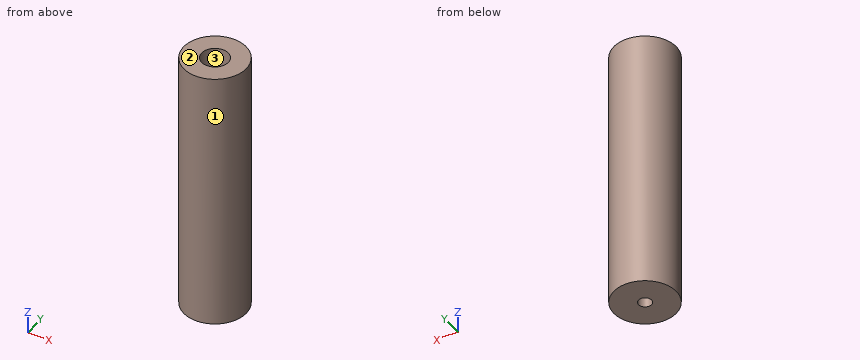
```python
from build123d import *

# Parameters (mm, degrees)
F0_R     = 5.95
F1_DEPTH = 50
F3_D     = 2.5
F4_R     = 2.55
F4_R_2   = 1.25
F5_DEPTH = 25


with BuildPart() as f1:
    # F0 (on Top) → F1 (new body)
    with BuildSketch(Plane.XY):
        Circle(F0_R)
    extrude(amount=F1_DEPTH)

    # F3 (through all)
    with Locations(Plane(origin=(0, 0, 0), x_dir=(1, 0, 0), z_dir=(0, 0, -1))):
        with Locations((0, 0)):
            Hole(F3_D / 2)

    # F4 (on face) → F5 (cut)
    with BuildSketch(Plane.XY.offset(50)):
        Circle(F4_R)
        Circle(F4_R_2, mode=Mode.SUBTRACT)
    extrude(amount=-F5_DEPTH, mode=Mode.SUBTRACT)


solid = f1.part
```
Source: CAD feature listing. Evaluate the final solid. Frame: model axes, mm. Face numbers are marked on the shaded views. Coordinates: 2 decimals unless noted, no trailing zeros. Write each loop counter-clockwise with the first axis right and the second up, starting at its lowest first coordinate (ties: lowest second). Pieces come first, ordered by that corner, then holes. Notation, with made-up numbers: (-35.75, 48) -> (-12.75, 48) arc R15 ccw to (-12.75, 74) -> close; hole circle Ø1 at (58, 78.5). An arc over 180 degrees is marked (long way). Return JSON: item names as keys, results as strings. Group by question number.
1) Section query C-C, the plane z = 7. Return loops of the section in (x, y), plus the area to 3 significant figures.
2) Section query B-B, the plane y = 0.5. Return loops of the section in (x, z).
3) Section query D-D, the plane x = 2. Return loops of the section in (y, z).
4) Contact query for flat-ended pins moving along their axis: P1, Ø1, axis at x = -2, z = 40.5, coming from the -Y side; P2, Ø2, axis at x = 0, y = 0, coming from the -Z side; P3, Ø4, axis at x = -3.5, z = 11, coming from the +Y side; P4, Ø2, axis at x = -2, z = 29, coming from the +Y side. Output: stop coordinate, or through.
5) Mould query, pull axis X, two halves, no side actions, for the marked faces 1, 2 and 3. Classes: +X half, -X half, draft (parallel to the pull), parting line (faces both ways), or undercut.
6) Ray query, line 1 along Y through (x, z) = (0, 15.5); line 2 along Y through (x, z) = (0, 40.25); line 3 along Z through (x, y) = (0.5, 1.5). Return the intervals inside material, ascending.
7) Section query A-A, the plane x = 0. Return loops of the section in (y, z), plus the area to 3 significant figures.
From the geometry:
{
 "1": {"outline": "circle Ø11.9 at (0, 0); hole circle Ø2.5 at (0, 0)", "area": "106 mm²"},
 "2": {"outline": "(-5.93, 0) -> (-1.15, 0) -> (-1.15, 25) -> (-2.5, 25) -> (-2.5, 50) -> (-5.93, 50) -> close; (1.15, 0) -> (5.93, 0) -> (5.93, 50) -> (2.5, 50) -> (2.5, 25) -> (1.15, 25) -> close"},
 "3": {"outline": "(-5.6, 0) -> (5.6, 0) -> (5.6, 50) -> (1.58, 50) -> (1.58, 25) -> (-1.58, 25) -> (-1.58, 50) -> (-5.6, 50) -> close"},
 "4": {"P1": "y = -5.76", "P2": "through", "P3": "y = 5.76", "P4": "y = 5.87"},
 "5": {"face 1": "parting line", "face 2": "draft", "face 3": "undercut"},
 "6": {"line 1": "-5.95 to -1.25, 1.25 to 5.95", "line 2": "-5.95 to -2.55, 2.55 to 5.95", "line 3": "0 to 25"},
 "7": {"outline": "(-5.95, 0) -> (-1.25, 0) -> (-1.25, 25) -> (-2.55, 25) -> (-2.55, 50) -> (-5.95, 50) -> close; (1.25, 0) -> (5.95, 0) -> (5.95, 50) -> (2.55, 50) -> (2.55, 25) -> (1.25, 25) -> close", "area": "405 mm²"}
}
